Part model, mm, in its own coordinate system. A direction names the side the tool comes from. Give positions to 0.01 mm unless a question says otherwise; leave off trailing zeros. Write each loop counter-clockwise with the first axis right and the second up, starting at its lowest first coordinate (ties: lowest second). Pieces come first, ordered by that corner, then holes. Notation, with made-up numbers: M 17,87.25 L 49,87.25 A14 ccw 49,101.25 Z; hole C 26.25,66 d2. An arc over 180 degrees is marked long. Answer as CSV lines item,"result". Start each with the question number.
Item 1: Two-plate mould, pull along X, no slides. Class faces 1 (the flat face through (17, -1, 2.775)), 2 (the flat face through (17, -1, 15.335)), 3 (the flat face through (0, -1, 9)), 4 (the flat face through (17, 0, 17)): +X half, -X half, draft (parallel to the pull), parting line (faces both ways), or undercut.
Item 2: Band-saw the part on B-B, the plane z = 7. List the corners of the cut face in (x, y).
Item 3: Pin check, flat tip, straight feed: pin 1 (2 mm diameter, centred on x = 17.5, z = 5.5, fed in from -Y). Stop position of the tip, or through.
Item 4: 3-axis set-ups, long thin cutter, end or side, ignore diameter. For faces 5 (the flat face through (17, -1, 0)), 6 (the flat face through (5.1, -1, 9)): which of +Z, -Z, +X, -X, +Y, -Y reach the whole face in a straight line?
Item 5: Wall check: L1, parallel to X at y = -0.7, z = 13.5; L2, parallel to Z at x = 32.57, y = -0.85 (3 decimals); L3, parallel to Z at x = 20, y = -0.3 (3 decimals). Give the ranges that are in metal, low to high. Write a range as from..to.
Item 6: Band-saw the part on A-A, the plane x = 24. List the corners of the cut face in (y, z) (3 decimals), then the cut area to 3 significant figures.
Item 7: Band-saw the part on C-C, the plane y = -0.6. List the corners of the cut face in (x, z) (3 decimals).
from build123d import *

# Parameters (mm, degrees)
SKETCH_W        = 35.12
SKETCH_H        = 18.11
PAD_DEPTH       = 2.6
SKETCH002_W     = 24.92
SKETCH002_H     = 12.56
POCKET_DEPTH    = 2.6
SKETCH003_R     = 0.5
SKETCH003_W     = 2.01
SKETCH003_H     = 3.5
POCKET001_DEPTH = 5


with BuildPart() as part:
    # Sketch → Pad (new body)
    with BuildSketch(Plane.XZ):
        with Locations((17.56, 9.055)):
            Rectangle(SKETCH_W, SKETCH_H)
    extrude(amount=PAD_DEPTH)

    # Sketch002 (on Face6 of Pad) → Pocket (cut)
    with BuildSketch(Plane.XZ.offset(2.6)):
        with Locations((17.56, 9.055)):
            Rectangle(SKETCH002_W, SKETCH002_H)
    extrude(amount=-POCKET_DEPTH, mode=Mode.SUBTRACT)

    # Sketch003 (on Face4 of Pocket) → Pocket001 (cut)
    with BuildSketch(Plane(origin=(0, 0, 0), x_dir=(1, 0, 0), z_dir=(0, 1, 0))):
        with Locations((32.57, -1.395)):
            Circle(SKETCH003_R)
        with Locations((27.953742, -8.544061)):
            Rectangle(SKETCH003_W, SKETCH003_H)
    extrude(amount=-POCKET001_DEPTH, mode=Mode.SUBTRACT)


solid = part.part
Output:
1,face 1,"undercut"
1,face 2,"undercut"
1,face 3,"-X half"
1,face 4,"draft"
2,outline,"M 0,-2.6 L 5.1,-2.6 L 5.1,0 L 0,0 Z; M 30.02,-2.6 L 35.12,-2.6 L 35.12,0 L 30.02,0 Z"
3,pin 1,"through"
4,face 5,"-Z, +X, -X, +Y, -Y"
4,face 6,"+Y, -Y"
5,L1,"0..5.1, 30.02..35.12"
5,L2,"0..0.895, 1.895..18.11"
5,L3,"0..2.775, 15.335..18.11"
6,outline,"M -2.6,0 L 0,0 L 0,2.775 L -2.6,2.775 Z; M -2.6,15.335 L 0,15.335 L 0,18.11 L -2.6,18.11 Z"
6,area,"14.4 mm²"
7,outline,"M 0,0 L 35.12,0 L 35.12,18.11 L 0,18.11 Z; hole M 5.1,2.775 L 30.02,2.775 L 30.02,15.335 L 5.1,15.335 Z; hole C 32.57,1.395 d1"
